```python
from build123d import *


with BuildPart() as f1:
    # F0 (on Top) → F1 (revolve)
    with BuildSketch(Plane.XY):
        with BuildLine():
            Line((-4.898979, 22), (-2.5, 22))
            Line((-2.5, 22), (-2.5, 0))
            Line((-2.5, 0), (-5, 0))
            Line((-5, 0), (-5, -1))
            ThreePointArc((-5, -1), (-2.7, -2.5), (0, -3))
            Line((0, -3), (0, 25))
            ThreePointArc((0, 25), (-2.645751, 24.480741), (-4.898979, 23))
            Line((-4.898979, 23), (-4.898979, 22))
        make_face()
    revolve(axis=Axis((0, 11, 0), (0, 1, 0)))


solid = f1.part
```
Read the model definition and answer for the solid it produces. Units are mm, in the model's axes. A direction names the side the tool comes from. Give positions to 0.01 mm unless a question says otherwise; leave off trailing zeros. Order: outer loops, then holes, each group sorted by start corner. A loop starts at its lowest first (then second) coordinate and runs counter-clockwise, first axis right, second up.
(1) For a pull along Y with two mould halves and no side action, classify faces 3 (the cylindrical face through (-4.673, 22.493, 1.472)), 4 (the cylindrical face through (0.54, 10.85, -2.44)) as released by +Y, released by -Y, zero draft, split by the parting line, or undercut.
(2) For faces 1 (the flat face through (-2, 22, -2)), 2 (the cylindrical face through (1.08, -0.51, -4.88)), determine the directions among +Z, -Z, +X, -X, +Y, -Y from which every point of the face is accessible in a straight line to the end or side of a thin tool.
(3) Straight lines are drawn through the part: L1, parallel to Y at x = -2.75, z = -0.5; L2, parallel to Y at x = 3.5, z = -1; L3, parallel to X at y = 20, z = -1. For each, find the intervals that lie inside material, in ascending order.
(4) Given pin 1 (4 mm diameter, centred on y = 19, z = 2.5, fed in from +X); pin 2 (4 mm diameter, centred on x = -2, z = 2.5, fed in from +Y); pin 3 (1 mm diameter, centred on x = 3.5, z = -1, fed in from +Y), each flat-ended and moving along its own axis, determine where each tip first touches the part or whether it passes through.
(5) Find section A-A (y = 4.5). Give the vertices of the cut face in (x, z).
Result sheet:
1. face 3: zero draft
1. face 4: undercut
2. face 1: none
2. face 2: +Y, -Y
3. L1: y = -2.46 to 0, 22 to 24.42
3. L2: y = -2.04 to 0, 22 to 23.98
3. L3: x = -2.29 to 2.29
4. pin 1: stops at x = 2.45
4. pin 2: stops at y = 24.9
4. pin 3: stops at y = 24.26
5. outline: circle Ø5 at (0, 0)
